```python
from build123d import *

# Parameters (mm, degrees)
ESBO_O1_W                = 77
ESBO_O1_H                = 135
RESSALTO_EXTRUS_O1_DEPTH = 3
ESBO_O4_W                = 3
ESBO_O4_H                = 21
CORTE_EXTRUS_O1_DEPTH    = 78.765673661
ESBO_O5_W                = 3
ESBO_O5_H                = 21
RESSALTO_EXTRUS_O2_DEPTH = 3
PADR_O_LINEAR1_COUNT     = 3
PADR_O_LINEAR1_PITCH     = 42


with BuildPart() as part:
    # Esboço1 → Ressalto-extrusão1 (new body)
    with BuildSketch(Plane.XY):
        Rectangle(ESBO_O1_W, ESBO_O1_H)
    extrude(amount=RESSALTO_EXTRUS_O1_DEPTH)

    # Esboço4 → Corte-extrusão1 (cut, through all)
    with BuildSketch(Plane.XY.offset(3)):
        with Locations((37, 42)):
            Rectangle(ESBO_O4_W, ESBO_O4_H)
        with Locations((37, 0)):
            Rectangle(ESBO_O4_W, ESBO_O4_H)
        with Locations((37, -42)):
            Rectangle(ESBO_O4_W, ESBO_O4_H)
    extrude(amount=-CORTE_EXTRUS_O1_DEPTH, mode=Mode.SUBTRACT)

    # Esboço5 → Ressalto-extrusão2 (add)
    with BuildSketch(Plane.XY.offset(3)):
        with Locations((-40, 42)):
            Rectangle(ESBO_O5_W, ESBO_O5_H)
    ressalto_extrus_o2 = extrude(amount=-RESSALTO_EXTRUS_O2_DEPTH)

    # Padrão linear1: Ressalto-extrusão2 ×3
    with Locations(*[(0, -i * PADR_O_LINEAR1_PITCH, 0) for i in range(1, PADR_O_LINEAR1_COUNT)]):
        add(ressalto_extrus_o2)


solid = part.part
```
Part model, mm, in its own coordinate system. A direction names the side the tool comes from. Round coordinates to 2 decimals unless told otherwise and drop trailing zeros. Order: outer loops, then holes, each group sorted by start corner. A loop starts at its lowest first (then second) coordinate and runs counter-clockwise, first axis right, second up. Notation, with made-up numbers: M -29,2 L 21,2 A6 cw 21,6 Z; hole C 50,69 d4. An arc over 180 degrees is marked long. Answer in a Markdown table with one row per item. Add a question column.
Q1. 3-axis set-ups, long thin cutter, end or side, ignore diameter. For faces 4 (the face through (38.5, 21, 1)), 5 (the face through (37, 10.5, 2)), 6 (the face through (-40, 31.5, 2)): which of +Z, -Z, +X, -X, +Y, -Y reach the whole face in a straight line?
Q2. Pin check, flat tips, straight feed: pin 1 (1.5 mm diameter, centred on x = -39.5, z = 1.5, fed in from -Y); pin 2 (0.9 mm diameter, centred on y = -37, z = 1.5, fed in from +X); pin 3 (1.5 mm diameter, centred on y = -63.5, z = 2, fed in from -X). Stop position of each tip, or through.
Q3. Cut at A-A on z = 0.6. Give the cut face in (x, y), and give its area (3 significant figures).
Q4. Wall check: L1, parallel to X at y = -48, z = 0.95; L2, parallel to X at y = 11, z = 0.95. Give the ranges that are in metal, low to high. Write a range as from..to.
Q5. Mould opens along Y. For faces 1 (the face through (-1, -67.5, 1)), 2 (the face through (-41.5, -42, 2)), 3 (the face through (37, 52.5, 2)) say: +Y half, -Y half, draft (parallel to the pull), parting line (faces both ways), or undercut.
Q6. Cut at B-B on y = 45.5. Give the cut face in (x, z), and give its area (3 significant figures).
Established:
| question | item | result |
|---|---|---|
| 1 | face 4 | +Z, -Z, +X, +Y, -Y |
| 1 | face 5 | +Z, -Z, +X |
| 1 | face 6 | +Z, -Z, -X |
| 2 | pin 1 | stops at y = -52.5 |
| 2 | pin 2 | stops at x = 35.5 |
| 2 | pin 3 | stops at x = -38.5 |
| 3 | outline | M -41.5,-52.5 L -38.5,-52.5 L -38.5,-67.5 L 38.5,-67.5 L 38.5,-52.5 L 35.5,-52.5 L 35.5,-31.5 L 38.5,-31.5 L 38.5,-10.5 L 35.5,-10.5 L 35.5,10.5 L 38.5,10.5 L 38.5,31.5 L 35.5,31.5 L 35.5,52.5 L 38.5,52.5 L 38.5,67.5 L -38.5,67.5 L -38.5,52.5 L -41.5,52.5 L -41.5,31.5 L -38.5,31.5 L -38.5,10.5 L -41.5,10.5 L -41.5,-10.5 L -38.5,-10.5 L -38.5,-31.5 L -41.5,-31.5 Z |
| 3 | area | 10,400 mm2 |
| 4 | L1 | x = -41.5..35.5 |
| 4 | L2 | x = -38.5..38.5 |
| 5 | face 1 | -Y half |
| 5 | face 2 | draft |
| 5 | face 3 | undercut |
| 6 | outline | M -41.5,0 L 35.5,0 L 35.5,3 L -41.5,3 Z |
| 6 | area | 231 mm2 |
